Source: CAD feature listing. Evaluate the final solid. Frame: model axes, mm. Face numbers are marked on the shaded views. A direction names the side the tool comes from. Give positions to 0.01 mm unless a question says otherwise; leave off trailing zeros. Write each loop counter-clockwise with the first axis right and the second up, starting at its lowest first coordinate (ties: lowest second). Pieces come first, ordered by that corner, then holes. Notation, with made-up numbers: M -36,12 L -14,12 A16 ccw -14,30 Z; hole C -5.5,89.25 d11. An arc over 180 degrees is marked long. Return JSON: item names as keys, results as strings.
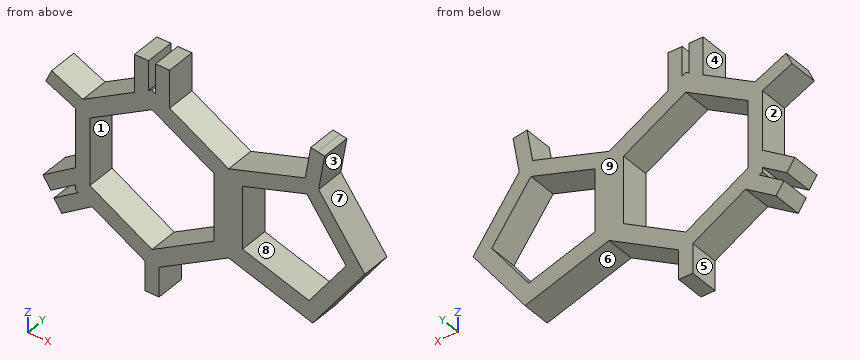
```python
from build123d import *

# Parameters (mm, degrees)
F1_DEPTH = 6.35
F3_DEPTH = 60.96


with BuildPart() as f1:
    # F0 (on Front) → F1 (new body)
    with BuildSketch(Plane.XZ):
        Polygon((0.762, 18.610059), (0, 19.05), (-0.710735, 18.639657), (-3.758735, 16.879893), (-14.88736, 10.454779), (-16.497784, 9.525), (-16.497784, 7.842908), (-16.497784, 0), (-16.497784, -4.870526), (-16.497784, -8.526968), (-16.497784, -9.525), (-15.84291, -9.903091), (-12.894138, -11.605566), (-1.524, -18.170118), (0, -19.05), (1.524, -18.170118), (16.497784, -9.525), (16.497784, 0), (16.497784, 9.525), (3.81, 16.850295), align=None)
        Polygon((0.762, 24.960059), (0.762, 18.610059), (3.81, 16.850295), (3.81, 24.960059), align=None)
        Polygon((-3.758735, 16.879893), (-0.710735, 18.639657), (-0.710735, 24.989657), (-3.758735, 24.989657), align=None)
        Polygon((32.980273, 14.880485), (16.497784, 9.525), (16.497784, 0), (16.497784, -9.525), (34.615411, -15.411774), (45.81272, 0), (35.869741, 13.685336), (34.615411, 15.411774), align=None)
        Polygon((-16.497784, 9.525), (-14.88736, 10.454779), (-21.605948, 13.593383), (-22.250976, 12.212617), (-22.896004, 10.831851), (-16.497784, 7.842908), align=None)
        Polygon((34.168763, 21.926801), (32.980273, 14.880485), (34.615411, 15.411774), (35.869741, 13.685336), (37.17431, 21.419861), (35.671536, 21.673331), align=None)
        Polygon((1.524, -24.520118), (1.524, -18.170118), (0, -19.05), (-1.524, -18.170118), (-1.524, -24.520118), (0, -24.520118), align=None)
        Polygon((-16.497784, -8.526968), (-16.497784, -4.870526), (-23.474759, -9.49373), (-21.791126, -12.034534), align=None)
        Polygon((-19.452621, -15.951463), (-12.894138, -11.605566), (-15.84291, -9.903091), (-21.136253, -13.410658), align=None)
    extrude(amount=F1_DEPTH)

    # F2 (on face) → F3 (cut)
    with BuildSketch(Plane.XZ):
        Polygon((13.382281, 7.118522), (0, 14.844785), (-13.382281, 7.118522), (-13.382281, -7.308772), (0, -15.035036), (13.382281, -7.308772), align=None)
        Polygon((19.496603, 7.118522), (19.496603, -6.312186), (33.812493, -10.9637), (41.778088, 0), (33.338541, 11.61604), align=None)
    extrude(amount=F3_DEPTH, mode=Mode.SUBTRACT)


solid = f1.part
```
1) Draft query along X for the marked faces 6, 7, 8 and 9. Return one class per face: released by +X, released by -X, zero draft, split by the parting line, or undercut.
Numbers:
{"face 6": "undercut", "face 7": "released by +X", "face 8": "undercut", "face 9": "zero draft"}
2) Cut plane D-D, the plane x = 21. Return the cut outline in (y, z), then the cut area to 3 significant figures.
Numbers:
{"outline": "M -6.35,-10.99 L 0,-10.99 L 0,-6.8 L -6.35,-6.8 Z; M -6.35,7.61 L 0,7.61 L 0,10.99 L -6.35,10.99 Z", "area": "48.1 mm²"}
3) Line query: line 1 (X direction, y = -2, z = 22); line 2 (Z direction, x = -20, y = -2.25); line 3 (X direction, y = -5.5, z = 3). Output: solid intervals per line, ascending. Write a range as [from, to].
Numbers:
{"line 1": "x = [-3.76, -0.71], [0.76, 3.81]", "line 2": "z = [-15.13, -12.66], [-10.85, -7.19], [9.48, 12.84]", "line 3": "x = [-16.5, -13.38], [13.38, 19.5], [39.6, 43.63]"}
4) Cut plane C-C, the plane y = -4.75. Give the number of separate pieces and of enclosed holes in the cut face, then the cut area to 3 significant figures.
Numbers:
{"separate pieces": "1", "enclosed holes": "2", "area": "776 mm²"}
5) Set-up query: the marked faces 1, 2, 3, 4 and 5. Return all of +Z, -Z, +X, -X, +Y, -Y with unobstructed straight access to the full face (end or side cutting, diameter ignored); none if empty.
Numbers:
{"face 1": "+Y, -Y", "face 2": "-X, +Y, -Y", "face 3": "+X, +Y, -Y", "face 4": "+Z, -X, +Y, -Y", "face 5": "-Z, -X, +Y, -Y"}
6) Cut plane A-A, the plane x = 38. Return the cut outline in (y, z).
Numbers:
{"outline": "M -6.35,-10.75 L 0,-10.75 L 0,-5.2 L -6.35,-5.2 Z; M -6.35,5.2 L 0,5.2 L 0,10.75 L -6.35,10.75 Z"}
7) Cut plane B-B, the plane z = 20. Return the cut outline in (x, y), then the cut area to 3 significant figures.
Numbers:
{"outline": "M -3.76,-6.35 L -0.71,-6.35 L -0.71,0 L -3.76,0 Z; M 0.76,-6.35 L 3.81,-6.35 L 3.81,0 L 0.76,0 Z; M 33.84,-6.35 L 36.93,-6.35 L 36.93,0 L 33.84,0 Z", "area": "58.3 mm²"}
8) Contact query for flat-ended pins moving along their axis: pin 1 Ø1.9 at (y, z) = (-2, 22) entering from -X; pin 2 Ø3 at (y, z) = (-3, -20.5) entering from -X; pin 3 Ø1.9 at (y, z) = (-3.5, -20.5) entering from +X. Output: stop coordinate, or through.
Numbers:
{"pin 1": "stops at x = -3.76", "pin 2": "stops at x = -1.52", "pin 3": "stops at x = 1.52"}
